```python
from build123d import *

# Parameters (mm, degrees)
SKETCH1_W           = 25.4
SKETCH1_H           = 38.1
SKETCH1_R           = 1.905
BOSS_EXTRUDE1_DEPTH = 1.27
SKETCH2_W           = 6.35
SKETCH2_H           = 7.62
SKETCH2_R           = 1.905
BOSS_EXTRUDE2_DEPTH = 2.54
FILLET1_R           = 6.35


with BuildPart() as part:
    # Sketch1 → Boss-Extrude1 (new, symmetric)
    with BuildSketch(Plane.XY):
        Rectangle(SKETCH1_W, SKETCH1_H)
        with Locations((-7.62, 13.97)):
            Circle(SKETCH1_R, mode=Mode.SUBTRACT)
        with Locations((-7.62, -13.97)):
            Circle(SKETCH1_R, mode=Mode.SUBTRACT)
        with Locations((7.62, -13.97)):
            Circle(SKETCH1_R, mode=Mode.SUBTRACT)
    extrude(amount=BOSS_EXTRUDE1_DEPTH, both=True)

    # Sketch2 → Boss-Extrude2 (add)
    with BuildSketch(Plane.XZ.offset(19.05)):
        with Locations((-15.875, 2.54)):
            Rectangle(SKETCH2_W, SKETCH2_H)
        with Locations(Location((-15.875, 3.81, 0), (0, 0, 270))):
            Circle(SKETCH2_R, mode=Mode.SUBTRACT)
    boss_extrude2 = extrude(amount=-BOSS_EXTRUDE2_DEPTH)

    # Mirror5: Boss-Extrude2 across plane
    add(boss_extrude2.mirror(Plane(origin=(0, 0, 0), x_dir=(0, 0, 1), z_dir=(1, 0, 0))))

    # Fillet1
    fillet1_edges = [part.edges().sort_by_distance(p)[0] for p in [
        (-12.7, -16.51, 0),
        (12.7, -16.51, 0),
    ]]
    fillet(fillet1_edges, radius=FILLET1_R - 0.0001)  # a hair under: the kernel refuses the full size


solid = part.part
```
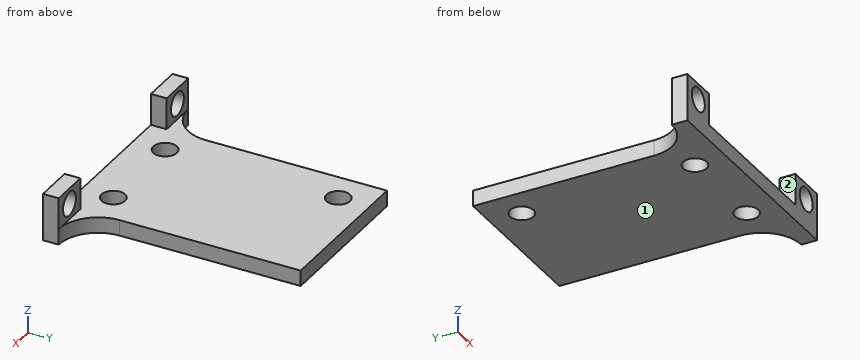
CAD build for the part. Positions are in the model's coordinates, mm. Face numbers are marked on the shaded views. Coordinates: 2 decimals unless noted, no trailing zeros. Order: outer loops, then holes, each group sorted by start corner. A loop starts at its lowest first (then second) coordinate and runs counter-clockwise, first axis right, second up.
(1) Saw through at B-B, the plane x = -7.62. Write the cut outline in (y, z) (3 decimals), and give its area (3 significant figures).
Solution:
outline: (-19.05, -1.27) - (-15.875, -1.27) - (-15.875, 1.27) - (-19.05, 1.27) - close; (-12.065, -1.27) - (12.065, -1.27) - (12.065, 1.27) - (-12.065, 1.27) - close; (15.875, -1.27) - (19.05, -1.27) - (19.05, 1.27) - (15.875, 1.27) - close
area: 77.4 mm2
(2) Saw through at C-C, the plane z = 3.81. Write the cut outline in (x, y).
Solution:
outline: (-19.05, -19.05) - (-17.78, -19.05) - (-17.78, -16.51) - (-19.05, -16.51) - close; (-13.97, -19.05) - (-12.7, -19.05) - (-12.7, -16.51) - (-13.97, -16.51) - close; (12.7, -19.05) - (13.97, -19.05) - (13.97, -16.51) - (12.7, -16.51) - close; (17.78, -19.05) - (19.05, -19.05) - (19.05, -16.51) - (17.78, -16.51) - close
(3) Saw through at D-D, the plane x = 7.62. Write the cut outline in (y, z) (3 decimals).
Solution:
outline: (-19.05, -1.27) - (-15.875, -1.27) - (-15.875, 1.27) - (-19.05, 1.27) - close; (-12.065, -1.27) - (19.05, -1.27) - (19.05, 1.27) - (-12.065, 1.27) - close
(4) Saw through at A-A, the plane y = 13.97. Write the cut outline in (x, z) (3 decimals), and give its area (3 significant figures).
Solution:
outline: (-12.7, -1.27) - (-9.525, -1.27) - (-9.525, 1.27) - (-12.7, 1.27) - close; (-5.715, -1.27) - (12.7, -1.27) - (12.7, 1.27) - (-5.715, 1.27) - close
area: 54.8 mm2
(5) Pin check, flat tips, straight feed: pin 1 Ø1.5 at (x, y) = (9, -5) entering from +Z; pin 2 Ø1.9 at (x, z) = (-15, 1.5) entering from +Y; pin 3 Ø6 at (x, y) = (7.62, -13.97) entering from -Z; pin 4 Ø3 at (y, z) = (-1, 0) entering from +X. Stop position of each tip, or through.
Solution:
pin 1: stops at z = 1.27
pin 2: stops at y = -14.11
pin 3: stops at z = -1.27
pin 4: stops at x = 12.7
(6) Drill centre lines: L1, parallel to X at y = -17.8, z = 3.81; L2, parallel to Y at x = 7.62, z = 0.6 (3 decimals); L3, parallel to Z at x = 5, y = 3.5. Where is each one in solid material? Low to high.
Solution:
L1: x = -19.05 to -17.78, -13.97 to -12.7, 12.7 to 13.97, 17.78 to 19.05
L2: y = -19.05 to -15.875, -12.065 to 19.05
L3: z = -1.27 to 1.27
(7) Mould opens along X. For the marked faces 1 and 2 say: released by +X, released by -X, zero draft, split by the parting line, or undercut.
Solution:
face 1: zero draft
face 2: undercut
